from build123d import *

# Parameters (mm, degrees)
PAD_DEPTH       = 114.3
SKETCH001_W     = 2.54
SKETCH001_H     = 12.7
POCKET_DEPTH    = 12.701
POCKET001_DEPTH = 12.701
CHAMFER_SIZE    = 3.81


with BuildPart() as part:
    # Sketch → Pad (new body)
    with BuildSketch(Plane.XY):
        with BuildLine():
            Line((0, 140.081), (12.7, 140.081))
            Line((12.7, 140.081), (12.7, 25.781))
            ThreePointArc((0, -28.739345), (27.989989, -6.520004), (12.7, 25.781))
            Line((0, -19.431), (0, -28.739345))
            ThreePointArc((0, -19.431), (19.431, 0), (0, 19.431))
            Line((0, 140.081), (0, 19.431))
        make_face()
    extrude(amount=PAD_DEPTH)

    # Sketch001 (on Face2 of Pad) → Pocket (cut, through all)
    with BuildSketch(Plane.YZ.offset(12.7)):
        with Locations((27.051, 12.7)):
            Rectangle(SKETCH001_W, SKETCH001_H)
        with Locations((27.051, 101.6)):
            Rectangle(SKETCH001_W, SKETCH001_H)
    extrude(amount=-POCKET_DEPTH, mode=Mode.SUBTRACT)

    # Sketch002 → Pocket001 (cut, through all)
    with BuildSketch(Plane.YZ.offset(12.7)):
        Polygon((63.881, 0), (140.081, 114.3), (140.081, 0), align=None)
    extrude(amount=-POCKET001_DEPTH, mode=Mode.SUBTRACT)

    # Chamfer
    chamfer_edges = [part.edges().sort_by_distance(p)[0] for p in [
        (6.35, 140.081, 114.3),
    ]]
    chamfer(chamfer_edges, length=CHAMFER_SIZE)


solid = part.part
CAD build for the part. Positions are in the model's coordinates, mm. A direction names the side the tool comes from. Round coordinates to 2 decimals unless told otherwise and drop trailing zeros. Order: outer loops, then holes, each group sorted by start corner. A loop starts at its lowest first (then second) coordinate and runs counter-clockwise, first axis right, second up. Notation, with made-up numbers: (63.25, 35) -> (102.25, 35) arc R27 ccw to (102.25, 63) -> close; hole circle Ø2 at (37.25, -27.75). An arc over 180 degrees is marked (long way). Write item = value, one per line. Start each with the question number.
(1) Cut at B-B, the plane y = 35. List the corners of the cut face in (x, z), then the cut area to 3 significant figures.
(2) Cut at D-D, the plane z = 42.5. List the corners of the cut face in (x, y), then the cut area to 3 significant figures.
(3) Which spindle directions (+Z, -Z, +X, -X, +Y, -Y) get a long thin tool onto all of the face, cutting with end or side? Do faces 5 (the flat face through (12.7, 70, 69)), 6 (the flat face through (6.261, 137.131, 112.693)), 7 (the flat face through (6, 28.321, 102)). Say none if no direction does.
(4) Probe line 1 (Y direction, x = 10.25, z = 10); line 2 (Y direction, x = 6.5, z = 13); line 3 (X direction, y = 61.5, z = 25.5). List the from-to ranges inside material, lowest first. Write a range as [from, to].
(5) Cut at A-A, the plane x = 4.75. List the corners of the cut face in (y, z).
(6) Pull direction Z, two halves, no side cores. Call faces 1 (the cylindrical face through (27.863, -7.045, 56.35)), 2 (the flat face through (6, 28.321, 13)), 3 (the flat face through (6, 25.781, 102)), 4 (the flat face through (6.44, 100.41, 54.79)): released by +Z, released by -Z, zero draft, split by the parting line, or undercut.
(7) Cut at C-C, the plane x = 15.5. List the corners of the cut face in (y, z).
(8) Pin check, flat tips, straight feed: P1, Ø12, axis at y = 60, z = 14, coming from the +X side; P2, Ø1.5, axis at x = 12.5, z = 61.5, coming from the -Y side; P3, Ø6, axis at x = 10, z = 16, coming from the +Y side. Stop position of each tip, or through.
Model answer:
q1.outline = (0, 0) -> (12.7, 0) -> (12.7, 114.3) -> (0, 114.3) -> close
q1.area = 1,450 mm2
q2.outline = (0, -28.74) arc R28.74 ccw to (12.7, 25.78) -> (12.7, 92.21) -> (0, 92.21) -> (0, 19.43) arc R19.43 cw to (0, -19.43) -> close
q2.area = 1,520 mm2
q3.face_5 = +Z, -Z, +X, +Y
q3.face_6 = +Z, +X, -X, +Y
q3.face_7 = +X, -X
q4.line_1 = [-26.85, -16.51], [16.51, 25.78], [28.32, 70.55]
q4.line_2 = [-27.99, -18.31], [18.31, 25.78], [28.32, 72.55]
q4.line_3 = [0, 12.7]
q5.outline = (-28.34, 0) -> (-18.84, 0) -> (-18.84, 114.3) -> (-28.34, 114.3) -> close; (18.84, 0) -> (63.88, 0) -> (137.97, 111.13) -> (136.27, 114.3) -> (18.84, 114.3) -> close; hole (25.78, 6.35) -> (28.32, 6.35) -> (28.32, 19.05) -> (25.78, 19.05) -> close; hole (25.78, 95.25) -> (28.32, 95.25) -> (28.32, 107.95) -> (25.78, 107.95) -> close
q6.face_1 = zero draft
q6.face_2 = undercut
q6.face_3 = undercut
q6.face_4 = released by -Z
q7.outline = (-24.2, 0) -> (-11.72, 0) -> (-11.72, 114.3) -> (-24.2, 114.3) -> close; (11.72, 0) -> (24.2, 0) -> (24.2, 114.3) -> (11.72, 114.3) -> close
q8.P1 = 12.7
q8.P2 = -26.23
q8.P3 = 76.55
